from build123d import *

# Parameters (mm, degrees)
F1_DEPTH = 5.842
F3_DEPTH = 25.4


with BuildPart() as f1:
    # F0 (on Front) → F1 (new body)
    with BuildSketch(Plane.XZ):
        Polygon((86.36, 6.35), (-190.5, 6.35), (-190.5, -6.35), (-5.08, -6.35), (-5.08, -19.05), (58.42, -19.05), (58.42, -6.35), (177.8, -6.35), (177.8, -12.7), (190.5, -12.7), (190.5, -6.35), (190.5, 6.35), (130.175, 6.35), (128.860199, 1.443097), (125.685199, 1.443097), (127, 6.35), (120.015, 6.35), (118.700199, 1.443097), (115.525199, 1.443097), (116.84, 6.35), (109.855, 6.35), (108.540199, 1.443097), (105.365199, 1.443097), (106.68, 6.35), (99.695, 6.35), (98.380199, 1.443097), (95.205199, 1.443097), (96.52, 6.35), (89.535, 6.35), (88.220199, 1.443097), (85.045199, 1.443097), align=None)
    extrude(amount=F1_DEPTH)

    # F2 (on face) → F3 (cut)
    with BuildSketch(Plane.XZ.offset(5.842)):
        Polygon((58.42, -19.05), (-5.08, -15.875), (-5.08, -19.05), align=None)
    extrude(amount=-F3_DEPTH, mode=Mode.SUBTRACT)


solid = f1.part
Input: part model. Units: mm. Frame: model coordinates. A direction names the side the tool comes from. Round coordinates to 2 decimals unless told otherwise and drop trailing zeros. Order: outer loops, then holes, each group sorted by start corner. A loop starts at its lowest first (then second) coordinate and runs counter-clockwise, first axis right, second up. Notation, with made-up numbers: (76, 18) - (126, 18) arc R28 cw to (126, 51) - close; hole circle Ø9 at (30.25, -33). An arc over 180 degrees is marked (long way). Answer as a JSON object with one key per item and string values. Group by question number.
(1) Cut plane C-C (x = 49.5). Return loops of the section in (y, z), then the cut area to 3 significant figures.
(2) Reachability of faces 4 (the face through (58.42, -3, -13)), 5 (the face through (-190.5, -3, 0)), 6 (the face through (161, -3, 6.35)), 7 (the face through (184, -3, -12.7)), 8 (the face through (-5.08, -3, -11)) from +Z, -Z, +X, -X, +Y, -Y: full face, straight path, thin tool, end or side. Return the list, or none.
(3) Material intervals for probe 1 along X at (y, z) = (-2.3, -10.25); probe 2 along Z at (x, y) = (-104, -1.25); probe 3 along Z at (x, y) = (117, -3.8), sorted ascending. Write a range as from..to.
(4) Pin query (flat end, axial travel): P1, Ø1.8, axis at y = -2, z = -11, coming from the -X side; P2, Ø1, axis at x = 128, y = -2.5, coming from the +Z side; P3, Ø3, axis at x = 92, y = -3, coming from the -Z side; P4, Ø3, axis at x = -13.5, z = -9.5, coming from the -Y side. Return the tip coordinate at first contact, or that it passes through.
(5) Cut plane B-B (x = -101). Return loops of the section in (y, z), then the cut area to 3 significant figures.
(6) Draft query along X for faces 1 (the face through (190.5, -3, -3)), 2 (the face through (93, -3, 6.35)), 3 (the face through (117, -3, -6.35)). Return one class per face: released by +X, released by -X, zero draft, split by the parting line, or undercut.
Here are the results:
{
 "1": {"outline": "(-5.84, -18.6) - (0, -18.6) - (0, 6.35) - (-5.84, 6.35) - close", "area": "146 mm^2"},
 "2": {"face 4": "-Z, +Y, -Y", "face 5": "+Z, -Z, -X, +Y, -Y", "face 6": "+Z, +X, -X, +Y, -Y", "face 7": "-Z, +X, +Y, -Y", "face 8": "-Z, -X, +Y, -Y"},
 "3": {"probe 1": "x = -5.08..58.42, 177.8..190.5", "probe 2": "z = -6.35..6.35", "probe 3": "z = -6.35..1.44"},
 "4": {"P1": "stops at x = -5.08", "P2": "stops at z = 1.44", "P3": "stops at z = -6.35", "P4": "passes through"},
 "5": {"outline": "(-5.84, -6.35) - (0, -6.35) - (0, 6.35) - (-5.84, 6.35) - close", "area": "74.2 mm^2"},
 "6": {"face 1": "released by +X", "face 2": "zero draft", "face 3": "undercut"}
}
